Design review of the part built by this model. Coordinates are the model's own, in mm. A direction names the side the tool comes from. Round coordinates to 2 decimals unless told otherwise and drop trailing zeros. Loops run counter-clockwise (first coordinate to the right, second up) from the corner with the lowest first, then second, coordinate; pieces in that order, holes last. Notation, with made-up numbers: (-22, 73.25) -> (-7, 73.25) arc R24 ccw to (-7, 99.25) -> close; hole circle Ø9 at (-6, -11.75). An arc over 180 degrees is marked (long way). Answer as CSV lines item,"result". Start each with the question number.
(1) Take a section at A-A, the plane z = -16.66. Write out the cut boundary in (x, y).
(2) Take a section at D-D, the plane y = 0. State how many separate pieces and enclosed holes the cut face has, and give its area (3 significant figures).
(3) For P1, Ø3, axis at y = 0, z = 16.66, coming from the +X side; P2, Ø1.4, axis at y = 0, z = 0, coming from the +X side; P3, Ø3, axis at y = -6, z = 2, coming from the +X side, all flat-tipped, find the tip position at first contact; note any pin that passes through.
(4) To check wall thickness, follow line 1 (Z direction, x = 1.25, y = 0); line 2 (Y direction, x = 2.3, z = -16.66); line 3 (Z direction, x = 3.6, y = 0). State the ranges of each line that lie inside material, in increasing order. Write a range as from..to.
(5) Take a section at B-B, the plane x = 4. Write out the cut boundary in (y, z).
(6) Take a section at C-C, the plane y = -10. Write out the cut boundary in (x, z), and give its area (3 significant figures).
(7) Machinability: for faces 4 (the face through (8, 3, 22)), 5 (the face through (5.21, 0.18, 11.27)), which of the approach directions +Z, -Z, +X, -X, +Y, -Y give a long, thin tool a straight path to every point of the face, cutting with its end or side? Answer none if there is none.
(8) Draft analysis for pull direction Y (two halves, no side actions). For faces 1 (the face through (5.29, 0.18, -11.23)), 2 (the face through (4.82, 2.77, -16.3)), 3 (the face through (7.3, -11.8, -24.4)), state which applies: +Y half, -Y half, draft (parallel to the pull), parting line (faces both ways), or undercut.
Solid Edge part; units mm, degrees
sketch "Sketch1" plane through (0, 0, 0) normal (0, -1, 0) x (1, 0, 0)
  line L0 (0, 25) -> (0, -25)
  line L1 (0, -25) -> (8, -25)
  line L2 (8, -25) -> (8, -10)
  line L3 (8, -10) -> (2.5, -12.5)
  line L4 (2.5, -12.5) -> (2.5, 12.5)
  line L5 (2.5, 12.5) -> (8, 10)
  line L6 (8, 10) -> (8, 25)
  line L7 (8, 25) -> (0, 25)
  dimension "D1" = 2.5
  dimension "D2" = 8
  dimension "D3" = 8
  dimension "D4" = 8
extrude "Ajout_matière_1" add sketch "Sketch1" along normal mid plane 25
hole "Perçage_2" at (8, 0, 16.66) direction (-1, 0, 0) diameter 5.2197 end up to next countersink diameter 11.1125 countersink angle 82
hole "Hole1" at (8, 0, -16.66) direction (-1, 0, 0) diameter 5.2197 end up to next countersink diameter 11.1125 countersink angle 82
sketch "Sketch2" plane through (2.5, 0, 0) normal (1, 0, 0) x (0, 1, 0)
  circle A0 centre (0, 0) radius 5
extrude "Enlèvement_matière_1" cut sketch "Sketch2" against normal blind 1
fillet "Congé_1" radius 10 1 edges at (1.5, -5, 0)
chamfer "Chanfrein_1" distance 1 angle 45 10 edges at (4, -12.5, 25) (8, 0, 25) (8, 12.5, 17.5) (8, -12.5, 17.5) (8, -12.5, -17.5) (8, 12.5, -17.5) (8, 0, -25) (4, -12.5, -25) (4, 12.5, -25) (4, 12.5, 25)
properties material "Aluminium AU4G, 2024_T4"
The answers:
1,outline,"(0, -12.5) -> (7, -12.5) -> (8, -11.5) -> (8, -5.56) -> (4.61, -2.61) -> (0, -2.61) -> close; (0, 2.61) -> (4.61, 2.61) -> (8, 5.56) -> (8, 11.5) -> (7, 12.5) -> (0, 12.5) -> close"
2,separate pieces,"3"
2,enclosed holes,"0"
2,area,"165 mm²"
3,P1,"through"
3,P2,"x = 1.5"
3,P3,"x = 2.5"
4,line 1,"-25..-19.27, -14.05..14.05, 19.27..25"
4,line 2,"-12.5..-2.61, 2.61..12.5"
4,line 3,"-25..-19.27, -14.05..-12, 12..14.05, 19.27..25"
5,outline,"(-12.5, -24) -> (-11.5, -25) -> (11.5, -25) -> (12.5, -24) -> (12.5, -11.82) -> (-12.5, -11.82) -> close; (-12.5, 11.82) -> (12.5, 11.82) -> (12.5, 24) -> (11.5, 25) -> (-11.5, 25) -> (-12.5, 24) -> close; hole circle Ø5.22 at (0, -16.66); hole circle Ø5.22 at (0, 16.66)"
6,outline,"(0, -25) -> (7, -25) -> (8, -24) -> (8, -10) -> (2.5, -12.5) -> (2.5, 12.5) -> (8, 10) -> (8, 24) -> (7, 25) -> (0, 25) -> close"
6,area,"275 mm²"
7,face 4,"+Z, -Z, +X, +Y, -Y"
7,face 5,"+Y, -Y"
8,face 1,"draft"
8,face 2,"undercut"
8,face 3,"-Y half"
